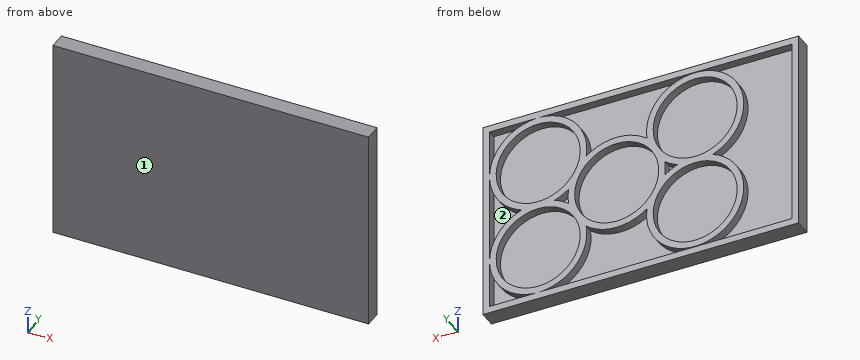
from build123d import *

# Parameters (mm, degrees)
SKETCH1_W           = 76.04
SKETCH1_H           = 48.67
BOSS_EXTRUDE1_DEPTH = 2
SKETCH2_R           = 10.115
BOSS_EXTRUDE5_DEPTH = 2
BOSS_EXTRUDE6_DEPTH = 2


with BuildPart() as part:
    # Sketch1 → Boss-Extrude1 (new body)
    with BuildSketch(Plane(origin=(0, 0, 0), x_dir=(1, 0, 0), z_dir=(0, 1, 0))):
        with Locations((-5.18381875, 15.397172461)):
            Rectangle(SKETCH1_W, SKETCH1_H)
    extrude(amount=BOSS_EXTRUDE1_DEPTH)

    # Sketch2 → Boss-Extrude5 (add)
    with BuildSketch(Plane(origin=(0, 2, 0), x_dir=(1, 0, 0), z_dir=(0, 1, 0))):
        with BuildLine():
            ThreePointArc((7.966863666, 24.51864889), (0.632329313, 27.112160631), (-6.709546926, 24.539506243))
            ThreePointArc((-6.709546926, 24.539506243), (-24.147153985, 36.457660066), (-22.544533536, 15.397172461))
            ThreePointArc((-22.544533536, 15.397172461), (-24.147153985, -5.663315144), (-6.709546926, 6.254838679))
            ThreePointArc((-6.709546926, 6.254838679), (0.632329313, 3.682184291), (7.966863666, 6.275696032))
            ThreePointArc((7.966863666, 6.275696032), (10.484956429, -3.077490534), (19.183945951, -7.337827539))
            Line((19.183945951, -7.337827539), (19.868416549, -7.337827539))
            ThreePointArc((19.868416549, -7.337827539), (27.809937192, -3.911583481), (31.23618125, 4.029937162))
            Line((31.23618125, 4.029937162), (31.23618125, 4.71440776))
            ThreePointArc((31.23618125, 4.71440776), (29.009139273, 11.250742962), (23.487317451, 15.397172461))
            ThreePointArc((23.487317451, 15.397172461), (29.009139273, 19.54360196), (31.23618125, 26.079937162))
            Line((31.23618125, 26.079937162), (31.23618125, 26.76440776))
            ThreePointArc((31.23618125, 26.76440776), (27.809937192, 34.705928403), (19.868416549, 38.132172461))
            Line((19.868416549, 38.132172461), (19.183945951, 38.132172461))
            ThreePointArc((19.183945951, 38.132172461), (10.484956429, 33.871835456), (7.966863666, 24.51864889))
        make_face()
        with Locations(Location((-18.289653985, 4.482172461, 0), (0, 0, 270))):
            Circle(SKETCH2_R, mode=Mode.SUBTRACT)
        with Locations(Location((0.61568058, 15.397172461, 0), (0, 0, 270))):
            Circle(SKETCH2_R, mode=Mode.SUBTRACT)
        with Locations(Location((19.52618125, 4.372172461, 0), (0, 0, 270))):
            Circle(SKETCH2_R, mode=Mode.SUBTRACT)
        with Locations(Location((-18.289653985, 26.312172461, 0), (0, 0, 270))):
            Circle(SKETCH2_R, mode=Mode.SUBTRACT)
        with BuildLine():
            ThreePointArc((-10.964426478, 17.169838679), (-11.09931942, 15.397172461), (-10.964426478, 13.624506243))
            ThreePointArc((-10.964426478, 13.624506243), (-12.432153985, 14.627660066), (-14.034774433, 15.397172461))
            ThreePointArc((-14.034774433, 15.397172461), (-12.432153985, 16.166684856), (-10.964426478, 17.169838679))
        make_face(mode=Mode.SUBTRACT)
        with BuildLine():
            ThreePointArc((12.174998164, 13.49364889), (12.33068058, 15.397172461), (12.174998164, 17.300696032))
            ThreePointArc((12.174998164, 17.300696032), (13.790504097, 16.207318933), (15.565045049, 15.397172461))
            ThreePointArc((15.565045049, 15.397172461), (13.790504097, 14.587025989), (12.174998164, 13.49364889))
        make_face(mode=Mode.SUBTRACT)
        with Locations(Location((19.52618125, 26.422172461, 0), (0, 0, 270))):
            Circle(SKETCH2_R, mode=Mode.SUBTRACT)
    extrude(amount=BOSS_EXTRUDE5_DEPTH)

    # Sketch3 → Boss-Extrude6 (add)
    with BuildSketch(Plane(origin=(0, 2, 0), x_dir=(1, 0, 0), z_dir=(0, 1, 0))):
        Polygon((-41.60381875, 39.732172461), (-43.20381875, 39.732172461), (-43.20381875, -8.937827539), (31.23618125, -8.937827539), (32.83618125, -8.937827539), (32.83618125, 39.732172461), align=None)
        Polygon((-41.60381875, -7.337827539), (-41.60381875, 38.132172461), (19.183945951, 38.132172461), (19.868416549, 38.132172461), (31.23618125, 38.132172461), (31.23618125, 26.76440776), (31.23618125, 26.079937162), (31.23618125, 4.71440776), (31.23618125, 4.029937162), (31.23618125, -7.337827539), (19.868416549, -7.337827539), (19.183945951, -7.337827539), align=None, mode=Mode.SUBTRACT)
    extrude(amount=BOSS_EXTRUDE6_DEPTH)


solid = part.part
Input: part model. Units: mm. Frame: model coordinates. Face numbers are marked on the shaded views. Coordinates: 2 decimals unless noted, no trailing zeros. Loops run counter-clockwise (first coordinate to the right, second up) from the corner with the lowest first, then second, coordinate; pieces in that order, holes last.
(1) Section B-B on z = 1.5. Return the cut outline in (x, y).
(2) Pull-direction query (X, two-part tool) for the marked faces 1 and 2; classes: released by +X, released by -X, zero draft, split by the parting line, or undercut.
(3) Section D-D on x = 28.5. Return the cut outline in (y, z), then the cut area to 3 significant figures.
(4) Section C-C on y = 3.1. Count the separate pieces of the cut face and the enclosed holes in it, then the cut area to 3 significant figures.
(5) First-contact query: pin 1 Ø23.5 at (x, z) = (19.53, -4.37) entering from +Y; pin 2 Ø5.5 at (x, z) = (23.5, -31.5) entering from +Y. Flat tips, straight axial feed; report the tip coordinate or a pass-through.
(6) Material intervals for probe 1 along Z at (x, y) = (1, 2.4); probe 2 along Z at (x, y) = (-35, 3.85); probe 3 along Z at (x, y) = (27, 3.2), sorted ascending.
(7) Section A-A on x = -36. Return the cut outline in (y, z).
Data:
1. outline: (-43.2, 0) - (32.84, 0) - (32.84, 4) - (31.24, 4) - (31.24, 2) - (29.66, 2) - (29.66, 4) - (27.76, 4) - (27.76, 2) - (11.29, 2) - (11.29, 4) - (9.39, 4) - (9.39, 2) - (-8.22, 2) - (-8.22, 4) - (-10.13, 4) - (-10.13, 2) - (-26.45, 2) - (-26.45, 4) - (-28.36, 4) - (-28.36, 2) - (-41.6, 2) - (-41.6, 4) - (-43.2, 4) - close
2. face 1: zero draft
2. face 2: undercut
3. outline: (0, -39.73) - (4, -39.73) - (4, -38.13) - (2, -38.13) - (2, -33.95) - (4, -33.95) - (4, -31.09) - (2, -31.09) - (2, -21.75) - (4, -21.75) - (4, -18.89) - (2, -18.89) - (2, -11.9) - (4, -11.9) - (4, -9.04) - (2, -9.04) - (2, 0.3) - (4, 0.3) - (4, 3.16) - (2, 3.16) - (2, 7.34) - (4, 7.34) - (4, 8.94) - (0, 8.94) - close
3. area: 127 mm2
4. separate pieces: 1
4. enclosed holes: 11
4. area: 885 mm2
5. pin 1: stops at y = 4
5. pin 2: stops at y = 2
6. probe 1: z = -39.73 to -38.13, -27.11 to -25.5, -5.29 to -3.69, 7.34 to 8.94
6. probe 2: z = -39.73 to -38.13, 7.34 to 8.94
6. probe 3: z = -39.73 to -38.13, -35.44 to -33.24, -19.61 to -17.4, -13.39 to -11.19, 2.44 to 4.65, 7.34 to 8.94
7. outline: (0, -39.73) - (4, -39.73) - (4, -38.13) - (2, -38.13) - (2, 7.34) - (4, 7.34) - (4, 8.94) - (0, 8.94) - close
